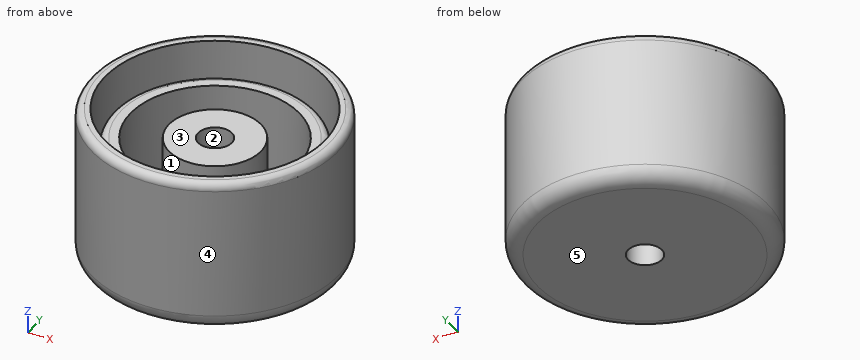
```python
from build123d import *

# Parameters (mm, degrees)
F0_R        = 6.6
F0_R_2      = 5.5
F1_DEPTH    = 6
F0_R_3      = 7.15
F0_R_4      = 3
F2_DEPTH    = 0.5
F0_R_5      = 8
F3_DEPTH    = 8
F0_R_6      = 1.1
F4_DEPTH    = 6
F5_R        = 0.5
F4_FACE_R   = 8
F4_FACE_R_2 = 1.1
F6_DEPTH    = 2
F7_R        = 1


with BuildPart() as f1:
    # F0 (on Top) → F1 (new body)
    with BuildSketch(Plane.XY):
        Circle(F0_R)
        Circle(F0_R_2, mode=Mode.SUBTRACT)
    extrude(amount=F1_DEPTH)

    # F0 (on Top) → F2 (join)
    with BuildSketch(Plane.XY):
        Circle(F0_R_3)
        Circle(F0_R, mode=Mode.SUBTRACT)
        Circle(F0_R_2)
        Circle(F0_R_4, mode=Mode.SUBTRACT)
    extrude(amount=F2_DEPTH)

    # F0 (on Top) → F3 (join)
    with BuildSketch(Plane.XY):
        Circle(F0_R_5)
        Circle(F0_R_3, mode=Mode.SUBTRACT)
    extrude(amount=F3_DEPTH)

    # F0 (on Top) → F4 (join)
    with BuildSketch(Plane.XY):
        Circle(F0_R_4)
        Circle(F0_R_6, mode=Mode.SUBTRACT)
    extrude(amount=F4_DEPTH)

    # F5
    f5_edges = [f1.edges().sort_by_distance(p)[0] for p in [
        (-6.6, 0, 6),
        (-8, 0, 8),
    ]]
    fillet(f5_edges, radius=F5_R)

    # F4_face (on face) → F6 (join)
    with BuildSketch(Plane(origin=(0, 0, 0), x_dir=(1, 0, 0), z_dir=(0, 0, -1))):
        Circle(F4_FACE_R)
        Circle(F4_FACE_R_2, mode=Mode.SUBTRACT)
    extrude(amount=F6_DEPTH)

    # F7
    f7_edges = [f1.edges().sort_by_distance(p)[0] for p in [
        (-8, 0, -2),
    ]]
    fillet(f7_edges, radius=F7_R)


solid = f1.part
```
Work out the finished part from the listing and answer in its coordinate system (mm). Face numbers are marked on the shaded views. A direction names the side the tool comes from. Round coordinates to 2 decimals unless told otherwise and drop trailing zeros. Order: outer loops, then holes, each group sorted by start corner. A loop starts at its lowest first (then second) coordinate and runs counter-clockwise, first axis right, second up.
Q1. Given pin 1 Ø3.5 at (x, y) = (0, 2.5) entering from +Z; pin 2 Ø1 at (x, z) = (4.5, 4.5) entering from -Y; pin 3 Ø2 at (y, z) = (5, 7) entering from +X, each flat-ended and moving along its own axis, determine where each tip first touches the part or whether it passes through.
Solution:
pin 1: stops at z = 6
pin 2: stops at y = -6.93
pin 3: stops at x = 6.93
Q2. The mould has two halves that part along X. Classify the marked faces 3, 4 and 5: pulls with the +X half, pulls with the -X half, needs draft (parallel to the pull), parting line crosses it, or undercut.
Solution:
face 3: undercut
face 4: parting line crosses it
face 5: needs draft
Q3. A cutting plane is placed at A-A, the plane z = 4.5. Determine the outline of the cut face in (x, y), then the cut area to 3 significant figures.
Solution:
outline: circle Ø16 at (0, 0); circle Ø13.2 at (0, 0); circle Ø6 at (0, 0); hole circle Ø14.3 at (0, 0); hole circle Ø11 at (0, 0); hole circle Ø2.2 at (0, 0)
area: 107 mm2
Q4. A tool of negligible diameter and unlimited length cuts with its end or side. For the marked faces 1 and 2, from which of +Z, -Z, +X, -X, +Y, -Y can it reach the whole face along a straight path? Write none if from no direction.
Solution:
face 1: +Z
face 2: +Z, -Z
Q5. Find the intervals of material crossed by line 1 along Y through (x, z) = (0, 3); line 2 along X through (y, z) = (-3.25, 5.5); line 3 along Y through (x, z) = (3.5, 4.25), in increasing order.
Solution:
line 1: y = -8 to -7.15, -6.6 to -5.5, -3 to -1.1, 1.1 to 3, 5.5 to 6.6, 7.15 to 8
line 2: x = -7.31 to -6.37, -5.74 to -4.44, 4.44 to 5.74, 6.37 to 7.31
line 3: y = -7.19 to -6.23, -5.6 to -4.24, 4.24 to 5.6, 6.23 to 7.19
